For this review, use the dimensioned drawing (mm, ordinates from the lowest corner) and the shaded views. A direction names the side the tool comes from. Coordinates: 2 decimals unless noted, no trailing zeros. Loops run counter-clockwise (first coordinate to the right, second up) from the corner with the lowest first, then second, coordinate; pieces in that order, holes last. Notation, with made-up numbers: M 4,73.25 L 33,73.25 A20 ccw 33,91.25 Z; hole C 10.5,14 d3. An arc over 180 degrees is marked long. One line per item, written item: value.
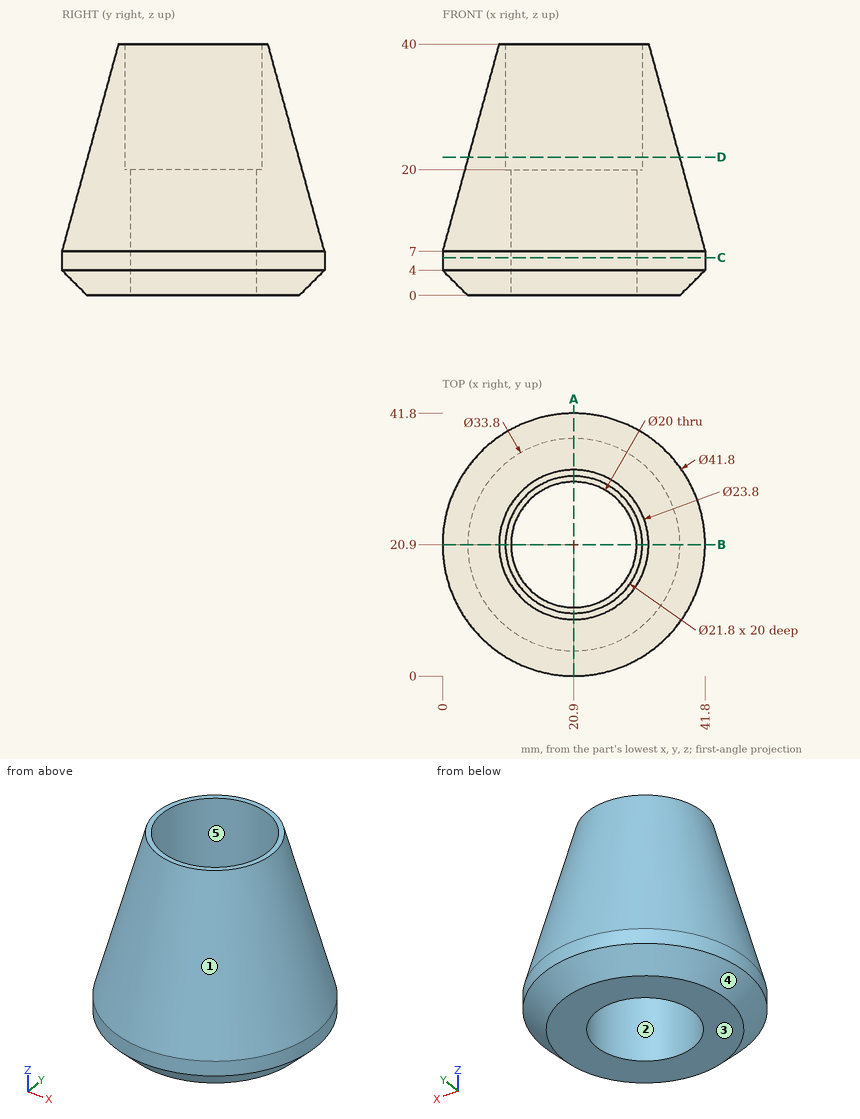
(1) Tool access review of the marked faces 4 and 5: name each direction out of +Z, -Z, +X, -X, +Y, -Y from which nothing blocks a thin tool from reaching the whole face with its end or side.
Reply:
face 4: -Z
face 5: +Z
(2) We need section C-C on z = 6. State the section outline as (x, y) points.
Reply:
outline: C 20.9,20.9 d41.8; hole C 20.9,20.9 d20
(3) Insertion check: pin 1 (2 mm diameter, centred on x = 18, z = 6.5, fed in from +Y); pin 2 (1 mm diameter, centred on x = 11.5, z = 28, fed in from -Y); pin 3 (1.5 mm diameter, centred on y = 14, z = 24.5, fed in from -X). Each pin has a flat end and moves straight along its axis. Give the tip position at first contact, or say it passes through.
Reply:
pin 1: stops at y = 41.71
pin 2: stops at y = 8.57
pin 3: stops at x = 5.92
(4) Mouldability with a two-part tool opening along Y and no side actions: class the marked faces 1, 2 and 3 as released by +Y, released by -Y, zero draft, split by the parting line, or undercut.
Reply:
face 1: split by the parting line
face 2: undercut
face 3: zero draft
(5) To check wall thickness, follow line 1 along X through (y, z) = (20.9, 6); line 2 along Y through (x, z) = (12, 16.5). State the ranges of each line that lie inside material, in increasing order. Write a range as [from, to].
Reply:
line 1: x = [0, 10.9], [30.9, 41.8]
line 2: y = [4.9, 16.34], [25.46, 36.9]
(6) We need section D-D on z = 22. State the section outline as (x, y) points.
Reply:
outline: C 20.9,20.9 d33.62; hole C 20.9,20.9 d21.8
(7) We need section A-A on x = 20.9. State the section outline as (y, z) points.
Reply:
outline: M 0,4 L 4,0 L 10.9,0 L 10.9,20 L 10,20 L 10,40 L 9,40 L 0,7 Z; M 30.9,0 L 37.8,0 L 41.8,4 L 41.8,7 L 32.8,40 L 31.8,40 L 31.8,20 L 30.9,20 Z
